```python
from build123d import *

# Parameters (mm, degrees)
F0_R     = 11.5
F1_DEPTH = 6
F2_COUNT = 3
F3_R     = 2


with BuildPart() as f1:
    # F0 (on Top) → F1 (new body)
    with BuildSketch(Plane.XY):
        with BuildLine():
            Line((15, -31.6162464206), (15, 0.3837535794))
            Line((15, 0.3837535794), (11.1837159736, 0.3837535794))
            ThreePointArc((11.1837159736, 0.3837535794), (-0.1936308108, -12.7913524315), (-11.5709775952, 0.3837535794))
            Line((-11.5709775952, 0.3837535794), (-15, 0.3837535794))
            Line((-15, 0.3837535794), (-15, -31.6162464206))
            ThreePointArc((-15, -31.6162464206), (0, -46.6162464206), (15, -31.6162464206))
        make_face()
        with Locations((0, -31.6162464206)):
            Circle(F0_R, mode=Mode.SUBTRACT)
    extrude(amount=F1_DEPTH)

    # F2: F1 ×3 about axis
    f2_axis = Axis((-0.1936308108, -1.2913524315, 0), (0, 0, -1))


with BuildPart() as f1_1:
    add(f1.part)
    for i in range(1, F2_COUNT):
        add(f1.part.rotate(f2_axis, i * 360 / F2_COUNT))

    # F3
    f3_edges = [f1_1.edges().sort_by_distance(p)[0] for p in [
        (8.945395, 21.52916, 6),
        (-24.526287, -4.78698, 6),
        (15, -20.616237, 6),
    ]]
    fillet(f3_edges, radius=F3_R)


solid = f1_1.part
```
Check sheet for the modelled part. Datum: model origin and axes. Units: mm. A direction names the side the tool comes from. Coordinates: 2 decimals unless noted, no trailing zeros. Order: outer loops, then holes, each group sorted by start corner. A loop starts at its lowest first (then second) coordinate and runs counter-clockwise, first axis right, second up. Notation, with made-up numbers: (-40, -14) -> (-5, -14) arc R20 cw to (-5, 22) -> close; hole circle Ø10 at (49, -30). An arc over 180 degrees is marked (long way). Write item = value, one per line. Start each with the question number.
1) Mould release check, pull along X, two halves, no side actions. Record for faces 1 (the cylindrical face through (8.59, 20.666, 5.399)), 2 (the cylindrical face through (-23.6, -4.66, 5.4)), 3 (the cylindrical face through (14.43, -19.88, 5.4)): +X half, -X half, draft (parallel to the pull), parting line (faces both ways), or undercut.
2) Go/stop test with flat-tipped pins: P1, Ø14, axis at x = 0, y = -31.62, coming from the -Z side; P2, Ø1.2, axis at y = -17, z = 2.5, coming from the -X side; P3, Ø3, axis at y = -1, z = 4, coming from the +X side; P4, Ø3, axis at x = 28.5, z = 2, coming from the +Y side. Record where each tip stops, or that it passes through.
3) Access from +Z, -Z, +X, -X, +Y, -Y to the whole of each face (thin tool, end or side, straight path). Record for faces 4 (the flat face through (-15, -21, 2)), 5 (the flat face through (15, -21, 2)), 6 (the cylindrical face through (-9.74, 20.66, 5.4)).
4) Material ranges on L1, parallel to X at y = 13.5, z = 3; L2, parallel to Y at x = -0.5, z = 4.5; L3, parallel to Y at x = 1.5, z = 5, recorded low to high.
5) Cross-section at A-A (z = 3). Enter the section's corners in (x, y).
6) Cross-section at B-B (y = -30.5). Enter the section's corners in (x, z).
Ans:
q1.face_1 = undercut
q1.face_2 = -X half
q1.face_3 = +X half
q2.P1 = through
q2.P2 = -15
q2.P3 = 32.52
q2.P4 = 29
q3.face_4 = +Z, -Z, -X, -Y
q3.face_5 = +Z, -Z, +X, -Y
q3.face_6 = +Z, +Y
q4.L1 = -41.55 to -38.05, -15.05 to 14.48, 37.46 to 40.96
q4.L2 = -46.54 to -43.11, -20.13 to -12.79, 10.2 to 16
q4.L3 = -46.27 to -43.02, -20.21 to -12.67, 10.08 to 16.92
q5.outline = (-34.05, 0.71) -> (-15, -10.29) -> (-15, -31.62) arc R15 ccw to (15, -31.62) -> (15, -9.62) -> (33.47, 1.05) arc R15 ccw to (18.47, 27.03) -> (-0.58, 16.03) -> (-19.05, 26.69) arc R15 ccw to start; hole circle Ø23 at (-26.55, 13.7); hole circle Ø23 at (-0.19, -1.29); hole circle Ø23 at (0, -31.62); hole circle Ø23 at (25.97, 14.04)
q6.outline = (-15, 0) -> (-11.45, 0) -> (-11.45, 6) -> (-13, 6) arc R2 ccw to (-15, 4) -> close; (11.45, 0) -> (15, 0) -> (15, 4) arc R2 ccw to (13, 6) -> (11.45, 6) -> close
